Autodesk Inventor part; units mm, degrees
ref_plane "Work Plane1" through (29, 0, 0) normal (0, -1, 0) x (1, 0, 0)
ref_plane "YZ Plane" through (0, 0, 0) normal (1, 0, 0) x (0, 1, 0)
ref_plane "XZ Plane" through (0, 0, 0) normal (0, 1, 0) x (-1, 0, 0)
sketch "Skizze1" plane through (0, 0, 0) normal (0, 0, 1) x (1, 0, 0)
  line L0 (-0.0667, 0) -> (35, 0)
  line L1 (35, 0) -> (35, 2)
  line L2 (35, 2) -> (15, 2)
  line L3 (15, 2) -> (14.5705, 2)
  line L4 (14.5705, 2) -> (0, 2)
  line L5 (0, 2) -> (0, 3.8)
  line L6 (0, 3.8) -> (-2.2, 3.8)
  line L7 (-2.2, 3.8) -> (-2.2, 1.4434)
  line L8 (-2.2, 1.4434) -> (-0.9, 1.4434)
  line L9 (-0.9, 1.4434) -> (-0.0667, 0)
  line L10 (-9.64, 0) -> (42.44, 0)
  line L11 (0, -0.76) -> (0, 4.56)
  line L12 (15, 2) -> (0, 2) construction
  dimension "d1" = 20
  dimension "d2" = 0.4295
  dimension "d3" = 2.2
  dimension "d4" = 1.3
  dimension "d5" = 60
  dimension "d6" = 4
  dimension "d7" = 4
  dimension "d8" = 2.8868
  dimension "d9" = 7.6
  dimension "d26" = 35
revolve "Körper" add sketch "Skizze1" angle 360 about axis through (-0.0667, 0, 0) along (1, 0, 0)
sketch "Skizze2" plane through (-2.2, 0, 0) normal (-1, 0, 0) x (0, 0, 1)
  circle A0 centre (0, 0) radius 1.4434
  line L0 (0, -5.32) -> (0, 5.32)
  line L1 (-5.32, 0) -> (5.32, 0)
  line L2 (1.4434, 0) -> (0.7217, -1.25)
  line L3 (0.7217, -1.25) -> (-0.7217, -1.25)
  line L4 (-0.7217, -1.25) -> (-1.4434, 0)
  line L5 (-1.4434, 0) -> (-0.7217, 1.25)
  line L6 (-0.7217, 1.25) -> (0.7217, 1.25)
  line L7 (0.7217, 1.25) -> (1.4434, 0)
extrude "Loch" add sketch "Skizze2" against normal up to next contours L7 A0 | A0 L2 | L6 L0 A0 | A0 L0 L3 | L0 L6 A0 | A0 L3 L0 | L4 A0 | A0 L5
fillet "Rundung1" radius 1.9 1 edges at (-2.2, -3.8, 0)
thread "Gewinde"
chamfer "Fase1" distance 0.4294 distance2 0.4294 1 edges at (35, -2, 0) measured on face at (35, 0.0262, -0.4421)
ref_plane "Work Plane1" through (29, 0, 0) normal (0, -1, 0) x (1, 0, 0)
fillet "Rundung2" radius 0.2 1 edges at (0, -2, 0)
equation "\"d1\" = GEL"
equation "\"d3\" = KOH"
equation "\"d4\" = INTI"
equation "\"d6\" = GD"
equation "\"d7\" = BDM"
equation "\"d8\" = 1.1547 * SW"
equation "\"d9\" = KOD"
equation "\"d26\" = NLG"
equation "\"d17\" = RR"
equation "\"d13\" = GEL"
equation "\"d15\" = -0.5 * SPD + 0.5 * GD"
equation "\"d16\" = GUL"
equation "\"d30\" = R"
equation "\"GD\" = NND"
equation "\"NLG\" = 35"
equation "\"GEL\" = 20"
equation "\"KOD\" = 7.6"
equation "\"KOH\" = 2.2"
equation "\"INTI\" = 1.3"
equation "\"GAL\" = 0.61345 * PTC"
equation "\"GUL\" = 0.61345 * PTC"
equation "\"BDM\" = NND"
equation "\"SW\" = 2.5"
equation "\"RR\" = 1.9"
equation "\"SPD\" = NND - 1.2269 * PTC"
equation "\"R\" = 0.2"
equation "\"TOA\" = 30deg"
equation "\"GD1\" = THREADDIA - 1.2269 * PTC"
equation "\"THREADDIA\" = 4"
equation "\"PTC\" = 0.7"
equation "\"NND\" = 4"
equation "\"KOH1\" = 0.3"
equation "\"E0\" = 2.873"
properties part number "ISO 7380-1 - M4 x 35" material "Stahl"
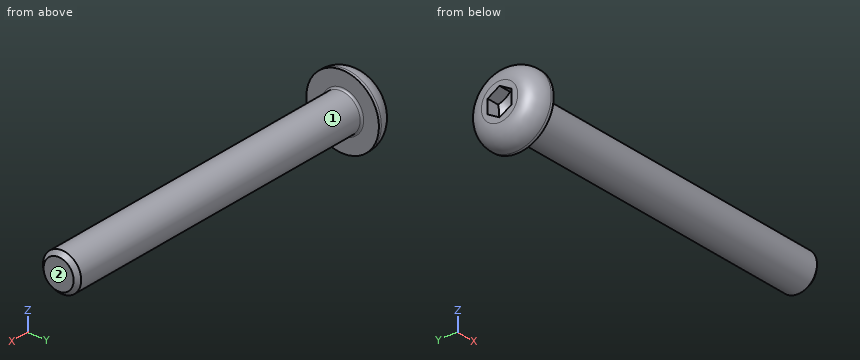
Work out the finished part from the listing and answer in its coordinate system (mm). Face numbers are marked on the shaded views. A direction names the side the tool comes from. Coordinates: 2 decimals unless noted, no trailing zeros. Write each loop counter-clockwise with the first axis right and the second up, starting at its lowest first coordinate (ties: lowest second). Pieces come first, ordered by that corner, then holes. Notation, with made-up numbers: (-15.5, 31.5) - (28.5, 31.5) arc R38 cw to (28.5, 69.5) - close; hole circle Ø4 at (-10.75, 29.5). An arc over 180 degrees is marked (long way). Answer as a JSON object with one key per item and string values.
Q1. Find section A-A (x = 23.5). Write down the section's boundary in (y, z).
Results list:
{"outline": "circle Ø4 at (0, 0)"}
Q2. Given pin 1 Ø1.5 at (x, y) = (26, 1) entering from -Z; pin 2 Ø2 at (x, z) = (27.5, 1) entering from -Y; pin 3 Ø2 at (y, z) = (-3, 2) entering from +X, each flat-ended and moving along its own axis, determine where each tip first touches the part or whether it passes through.
Results list:
{"pin 1": "stops at z = -1.98", "pin 2": "stops at y = -2", "pin 3": "stops at x = 0"}
Q3. Consider L1, parallel to Z at x = 8.5, y = 0; L2, parallel to X at y = 2.5, z = -2; L3, parallel to Y at x = 18, z = -1.25. Determine where each line is inside the solid, lowest interval first. Write a range as from..to.
Results list:
{"L1": "z = -2..2", "L2": "x = -1.68..0", "L3": "y = -1.56..1.56"}
Q4. Which of the six approach directions +Z, -Z, +X, -X, +Y, -Y give full straight-line access (tool end or side, diameter ignored) to the marked faces 1 and 2?
Results list:
{"face 1": "+X", "face 2": "+Z, -Z, +X, +Y, -Y"}
